```python
from build123d import *

# Parameters (mm, degrees)
BOSS_EXTRUDE2_DEPTH = 0.79375
CIRPATTERN1_COUNT   = 6


with BuildPart() as part:
    # Sketch1 → Revolve1 (revolve)
    with BuildSketch(Plane(origin=(0, 0, 0), x_dir=(1, 0, 0), z_dir=(0, 1, 0))):
        Polygon((-250, 0), (-150, 0), (-1, -22.35), (0, -22.35), (0, -17.5), (-150, 5), (-250, 5), align=None)
    revolve1 = revolve(axis=Axis((0, 0, 22.5), (-1, 0, 0)))

    # Sketch3 → Boss-Extrude2 (add, symmetric)
    with BuildSketch(Plane(origin=(0, 0, 0), x_dir=(1, 0, 0), z_dir=(0, 1, 0))):
        Polygon((-152, 14.3), (-158.141509434, 5), (-150, 5), (0, -17.5), (0, 14.3), align=None)
        Polygon((-158.141509434, 5), (-159.462264151, 3), (-150.149165611, 3), (-13.482498944, -17.5), (0, -17.5), (-150, 5), align=None)
    boss_extrude2 = extrude(amount=BOSS_EXTRUDE2_DEPTH, both=True)

    # CirPattern1: Revolve1, Boss-Extrude2 ×6 about axis
    cirpattern1_axis = Axis((0, 0, 22.5), (1, 0, 0))
    add([revolve1.rotate(cirpattern1_axis, i * 360 / CIRPATTERN1_COUNT) for i in range(1, CIRPATTERN1_COUNT)])
    add([boss_extrude2.rotate(cirpattern1_axis, i * 360 / CIRPATTERN1_COUNT) for i in range(1, CIRPATTERN1_COUNT)])


solid = part.part
```
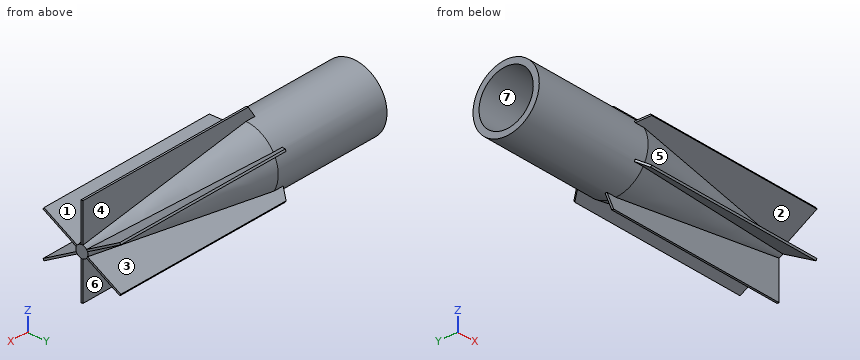
Part model, mm, in its own coordinate system. Face numbers are marked on the shaded views. A direction names the side the tool comes from. Round coordinates to 2 decimals unless told otherwise and drop trailing zeros. Order: outer loops, then holes, each group sorted by start corner. A loop starts at its lowest first (then second) coordinate and runs counter-clockwise, first axis right, second up. Notation, with made-up numbers: M -15,27.25 L 29,27.25 A12 ccw 29,36.25 Z; hole C 28,84 d3. An arc over 180 degrees is marked long. Answer in a Markdown table with one row per item. Add a question column.
Q1. Wall check: L1, parallel to Y at x = -0.2, z = 22.5; L2, parallel to Y at x = -121.5, z = 3.5; L3, parallel to Y at x = -48.5, z = 12.5. Give the ranges that are in metal, low to high. Write a range as from..to.
Q2. Cut at A-A on x = -31. Give the cut face in (y, z), and give its area (3 significant figures).
Q3. Pin check, flat tips, straight feed: pin 1 (1.5 mm diameter, centred on x = -162.5, z = 35, fed in from +Y); pin 2 (9.5 mm diameter, centred on x = -40, z = 45, fed in from +Y) (3 decimals); pin 3 (2 mm diameter, centred on x = -135.5, z = 21.5, fed in from -Y). Stop position of each tip, or through.
Q4. Cut at B-B on x = -167. Give the cut face in (y, z).
Q5. Mould opens along Y. For the marked faces 1, 2 and 3 say: +Y half, -Y half, draft (parallel to the pull), parting line (faces both ways), or undercut.
Q6. 3-axis set-ups, long thin cutter, end or side, ignore diameter. For the marked faces 4, 5, 6 and 7: which of +Z, -Z, +X, -X, +Y, -Y reach the whole face in a straight line?
Established:
| question | item | result |
|---|---|---|
| 1 | L1 | y = -5.03..-0.15, 0.15..5.03 |
| 1 | L2 | y = -31.52..-31.32, -13.36..13.36, 31.32..31.52 |
| 1 | L3 | y = -18.91..-15.73, -7.12..7.12, 15.73..18.91 |
| 2 | outline | M -32.27,4.79 L -31.47,3.41 L -7.93,17 A9.65 ccw -0.79,12.88 L -0.79,-14.3 L 0.79,-14.3 L 0.79,12.88 A9.65 ccw 7.93,17 L 31.47,3.41 L 32.27,4.79 L 8.73,18.38 A9.65 ccw 8.73,26.62 L 32.27,40.21 L 31.47,41.59 L 7.93,28 A9.65 ccw 0.79,32.12 L 0.79,59.3 L -0.79,59.3 L -0.79,32.12 A9.65 ccw -7.93,28 L -31.47,41.59 L -32.27,40.21 L -8.73,26.62 A9.65 ccw -8.73,18.38 Z; hole C 0,22.5 d9.3 |
| 2 | area | 483 mm2 |
| 3 | pin 1 | stops at y = 24.86 |
| 3 | pin 2 | stops at y = 32.245 |
| 3 | pin 3 | stops at y = -25.46 |
| 4 | outline | C 0,22.5 d55; hole C 0,22.5 d45 |
| 5 | face 1 | undercut |
| 5 | face 2 | -Y half |
| 5 | face 3 | +Y half |
| 6 | face 4 | +Z, +X |
| 6 | face 5 | +X, -Y |
| 6 | face 6 | -Z, +X |
| 6 | face 7 | -X |
